Geometry: see drawing. Coordinates: mm, zero at the bounding-box minimum. Coordinates: 2 decimals unless noted, no trailing zeros. Write each loop counter-clockwise with the first axis right and the second up, starting at its lowest first coordinate (ties: lowest second). Pieces come first, ordered by that corner, then holes. Notation, with made-up numbers: (65.5, -5) - (111.5, -5) arc R15 cw to (111.5, 8) - close; hole circle Ø4 at (55.5, 52). An arc over 180 degrees is marked (long way). Use a Markdown table: item, result. Add a question column.
Q1. Pin query (flat end, axial travel): P1, Ø2.5, axis at x = 49, y = 1.5, coming from the -Z side. Return the tip coordinate at first contact, or that it passes through.
Q2. Section query B-B (y = 4). Give the number of separate pieces and of enclosed holes in the cut face, then the cut area to 3 significant figures.
Q3. Material intervals for probe 1 along Z at (x, y) = (92.5, 4.85); probe 2 along X at (y, z) = (3.8, 28.25); probe 3 along X at (y, z) = (3.7, 16), sorted ascending. Write a range as from..to.
Q4. Section query A-A (x = 4.25). Return the cut outline in (y, z).
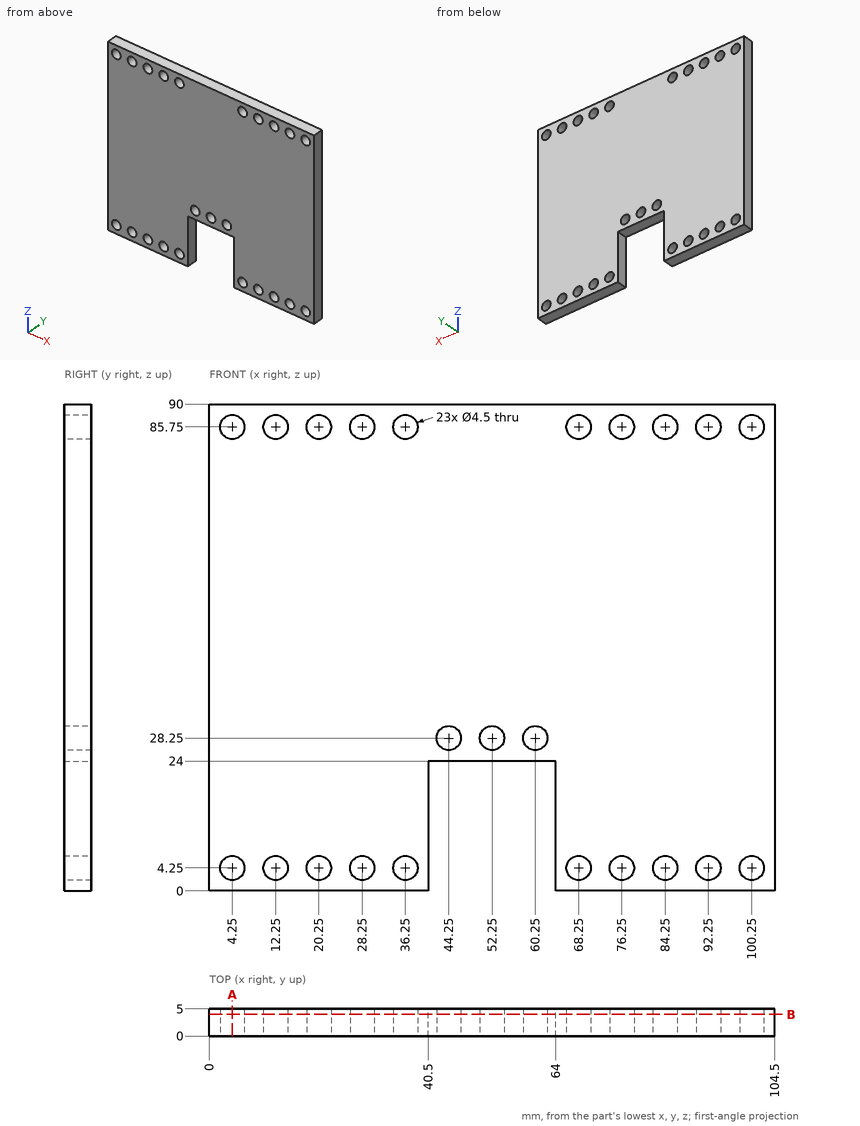
Values follow:
| question | item | result |
|---|---|---|
| 1 | P1 | z = 24 |
| 2 | separate pieces | 1 |
| 2 | enclosed holes | 23 |
| 2 | area | 8,480 mm2 |
| 3 | probe 1 | 0..2.01, 6.49..83.51, 87.99..90 |
| 3 | probe 2 | 0..42, 46.5..50, 54.5..58, 62.5..104.5 |
| 3 | probe 3 | 0..40.5, 64..104.5 |
| 4 | outline | (0, 0) - (5, 0) - (5, 2) - (0, 2) - close; (0, 6.5) - (5, 6.5) - (5, 83.5) - (0, 83.5) - close; (0, 88) - (5, 88) - (5, 90) - (0, 90) - close |
